Read the model definition and answer for the solid it produces. Units are mm, in the model's axes. A direction names the side the tool comes from. Round coordinates to 2 decimals unless told otherwise and drop trailing zeros. Write each loop counter-clockwise with the first axis right and the second up, starting at its lowest first coordinate (ties: lowest second). Pieces come first, ordered by that corner, then holes. Notation, with made-up numbers: (67, 6) - (76, 6) arc R6 cw to (76, 12) - close; hole circle Ø2 at (-29.75, 71). An arc over 180 degrees is marked (long way). Use one line per item in the form item = value. Start each with the question number.
1) For a pull along Z with two mould halves and no side action, classify faces 1 (the face through (-21.5, 6, 28)), 2 (the face through (-0.3, 2.7, 75)), 3 (the face through (-18, 5, 25.83)), 4 (the face through (0, 2, -50.44)) as released by +Z, released by -Z, zero draft, split by the parting line, or undercut.
2) The part is cut by section B-B, the plane z = -28.19. Give the vertices of the cut face in (x, y).
3) Each of these flat-tipped pins is pushed along its axis until it touches: pin 1 (1.5 mm diameter, centred on x = 18, y = 17.5, fed in from +Z); pin 2 (3 mm diameter, centred on x = 4, y = 5, fed in from -Z); pin 3 (6 mm diameter, centred on x = -8, z = -56.5, fed in from +Y); pin 4 (8 mm diameter, centred on x = -1, z = -23, fed in from +Y). Where does it stop, or does it pass through?
4) The part is cut by section A-A, the plane y = 12. Give the vertices of the cut face in (x, z), plus the area to 3 significant figures.
5) The part is cut by section C-C, the plane z = 70. Give the vertices of the cut face in (x, y).
6) Consider line 1 along X through (y, z) = (5.3, 30.83); line 2 along X through (y, z) = (1, 30.83); line 3 along X through (y, z) = (1, -28.19). Determine where each line is inside the solid, lowest interval first. Write a range as from..to.
7) For faces 5 (the face through (-19.325, 0.986, 33.211)), 6 (the face through (9, 0, -1)), 7 (the face through (8.15, 5, 32)), 8 (the face through (5, 5, 36.33)), determine the directions among +Z, -Z, +X, -X, +Y, -Y from which every point of the face is accessible in a straight line to the end or side of a thin tool.
8) The part is cut by section D-D, the plane x = 12. Give the vertices of the cut face in (y, z), plus the area to 3 significant figures.
from build123d import *

# Parameters (mm, degrees)
SKETCH1_W           = 43
SKETCH1_H           = 150
BOSS_EXTRUDE1_DEPTH = 3
SKETCH2_R           = 1.75
CUT_EXTRUDE1_DEPTH  = 10
SKETCH3_W           = 15
SKETCH3_H           = 75
CUT_EXTRUDE2_DEPTH  = 10
SKETCH4_W           = 5
SKETCH4_H           = 12
SKETCH4_W_2         = 4.116849784
SKETCH4_H_2         = 1.5
SKETCH4_H_3         = 3.5
BOSS_EXTRUDE2_DEPTH = 4
SKETCH5_W           = 8
SKETCH5_H           = 49.17
BOSS_EXTRUDE3_DEPTH = 4
SKETCH7_W           = 0.35
SKETCH7_H           = 12
BOSS_EXTRUDE4_DEPTH = 4
SKETCH8_R           = 1.75
CUT_EXTRUDE3_DEPTH  = 79.334219853
SKETCH9_W           = 5
SKETCH9_H           = 28
BOSS_EXTRUDE5_DEPTH = 15
SKETCH10_R          = 3
CUT_EXTRUDE5_DEPTH  = 2


with BuildPart() as part:
    # Sketch1 → Boss-Extrude1 (new body)
    with BuildSketch(Plane(origin=(0, 0, 0), x_dir=(1, 0, 0), z_dir=(0, 1, 0))):
        Rectangle(SKETCH1_W, SKETCH1_H)
    extrude(amount=BOSS_EXTRUDE1_DEPTH)

    # Sketch2 → Cut-Extrude1 (cut)
    with BuildSketch(Plane(origin=(0, 3, 0), x_dir=(1, 0, 0), z_dir=(0, 1, 0))):
        with Locations(Location((15.25, 28.19, 0), (0, 0, 270))):
            Circle(SKETCH2_R)
        with Locations(Location((-15.25, 28.19, 0), (0, 0, 270))):
            Circle(SKETCH2_R)
        with Locations(Location((-15.25, -2.31, 0), (0, 0, 270))):
            Circle(SKETCH2_R)
        with Locations(Location((15.25, -2.31, 0), (0, 0, 270))):
            Circle(SKETCH2_R)
    extrude(amount=-CUT_EXTRUDE1_DEPTH, mode=Mode.SUBTRACT)

    # Sketch3 → Cut-Extrude2 (cut)
    with BuildSketch(Plane(origin=(0, 3, 0), x_dir=(1, 0, 0), z_dir=(0, 1, 0))):
        with Locations((0, 12.94)):
            Rectangle(SKETCH3_W, SKETCH3_H)
    extrude(amount=-CUT_EXTRUDE2_DEPTH, mode=Mode.SUBTRACT)

    # Sketch4 → Boss-Extrude2 (add)
    with BuildSketch(Plane(origin=(0, 3, 0), x_dir=(1, 0, 0), z_dir=(0, 1, 0))):
        with Locations((-5.35, -31.83)):
            Rectangle(SKETCH4_W, SKETCH4_H)
        with Locations((10.65, -31.83)):
            Rectangle(SKETCH4_W, SKETCH4_H)
        with Locations((4.708424892, -37.08)):
            Rectangle(SKETCH4_W_2, SKETCH4_H_2)
        with Locations((4.708424892, -39.58)):
            Rectangle(SKETCH4_W_2, SKETCH4_H_3)
    extrude(amount=BOSS_EXTRUDE2_DEPTH)

    # Sketch5 → Boss-Extrude3 (add)
    with BuildSketch(Plane(origin=(0, 3, 0), x_dir=(1, 0, 0), z_dir=(0, 1, 0))):
        with Locations((-17.5, -50.415)):
            Rectangle(SKETCH5_W, SKETCH5_H)
        with Locations((17.5, -50.415)):
            Rectangle(SKETCH5_W, SKETCH5_H)
    extrude(amount=BOSS_EXTRUDE3_DEPTH)

    # Sketch7 → Boss-Extrude4 (add)
    with BuildSketch(Plane(origin=(0, 3, 0), x_dir=(1, 0, 0), z_dir=(0, 1, 0))):
        with Locations((13.325, -31.83)):
            Rectangle(SKETCH7_W, SKETCH7_H)
    extrude(amount=BOSS_EXTRUDE4_DEPTH)

    # Sketch8 → Cut-Extrude3 (cut, through all)
    with BuildSketch(Plane(origin=(0, 7, 0), x_dir=(1, 0, 0), z_dir=(0, 1, 0))):
        with Locations(Location((17.5, -70, 0), (0, 0, 270))):
            Circle(SKETCH8_R)
        with Locations(Location((17.5, -30.83, 0), (0, 0, 90))):
            Circle(SKETCH8_R)
        with Locations(Location((-17.5, -70, 0), (0, 0, 90))):
            Circle(SKETCH8_R)
        with Locations(Location((-17.5, -30.83, 0), (0, 0, 270))):
            Circle(SKETCH8_R)
    extrude(amount=-CUT_EXTRUDE3_DEPTH, mode=Mode.SUBTRACT)

    # Sketch9 → Boss-Extrude5 (add)
    with BuildSketch(Plane(origin=(0, 7, 0), x_dir=(1, 0, 0), z_dir=(0, 1, 0))):
        with Locations((19, -50.41)):
            Rectangle(SKETCH9_W, SKETCH9_H)
        with Locations((-19, -50.41)):
            Rectangle(SKETCH9_W, SKETCH9_H)
    extrude(amount=BOSS_EXTRUDE5_DEPTH)

    # Sketch10 → Cut-Extrude5 (cut)
    with BuildSketch(Plane.XZ):
        with Locations(Location((-17.5, 70, 0), (0, 0, 270))):
            Circle(SKETCH10_R)
        with Locations(Location((-17.5, 30.83, 0), (0, 0, 270))):
            Circle(SKETCH10_R)
        with Locations(Location((17.5, 30.83, 0), (0, 0, 270))):
            Circle(SKETCH10_R)
        with Locations(Location((17.5, 70, 0), (0, 0, 270))):
            Circle(SKETCH10_R)
    extrude(amount=-CUT_EXTRUDE5_DEPTH, mode=Mode.SUBTRACT)


solid = part.part
Geometry results:
q1.face_1 = zero draft
q1.face_2 = released by +Z
q1.face_3 = released by -Z
q1.face_4 = undercut
q2.outline = (-21.5, 0) - (-17, 0) - (-17, 3) - (-21.5, 3) - close; (-13.5, 0) - (-7.5, 0) - (-7.5, 3) - (-13.5, 3) - close; (7.5, 0) - (13.5, 0) - (13.5, 3) - (7.5, 3) - close; (17, 0) - (21.5, 0) - (21.5, 3) - (17, 3) - close
q3.pin_1 = 64.41
q3.pin_2 = 36.33
q3.pin_3 = 3
q3.pin_4 = through
q4.outline = (-21.5, 36.41) - (-16.5, 36.41) - (-16.5, 64.41) - (-21.5, 64.41) - close; (16.5, 36.41) - (21.5, 36.41) - (21.5, 64.41) - (16.5, 64.41) - close
q4.area = 280 mm2
q5.outline = (-21.5, 0) - (-20.5, 0) - (-20.5, 2) - (-19.25, 2) - (-19.25, 7) - (-21.5, 7) - close; (-15.75, 2) - (-14.5, 2) - (-14.5, 0) - (14.5, 0) - (14.5, 2) - (15.75, 2) - (15.75, 7) - (13.5, 7) - (13.5, 3) - (-13.5, 3) - (-13.5, 7) - (-15.75, 7) - close; (19.25, 2) - (20.5, 2) - (20.5, 0) - (21.5, 0) - (21.5, 7) - (19.25, 7) - close
q6.line_1 = -21.5..-19.25, -15.75..-13.5, -7.85..-2.85, 8.15..15.75, 19.25..21.5
q6.line_2 = -21.5..-20.5, -14.5..14.5, 20.5..21.5
q6.line_3 = -21.5..-17, -13.5..-7.5, 7.5..13.5, 17..21.5
q7.face_5 = -Y
q7.face_6 = +Z, -Z, +X, -X, -Y
q7.face_7 = +Z, -Z, +Y
q7.face_8 = -Z, +Y
q8.outline = (0, -75) - (3, -75) - (3, 25.83) - (7, 25.83) - (7, 37.83) - (3, 37.83) - (3, 75) - (0, 75) - close
q8.area = 498 mm2
